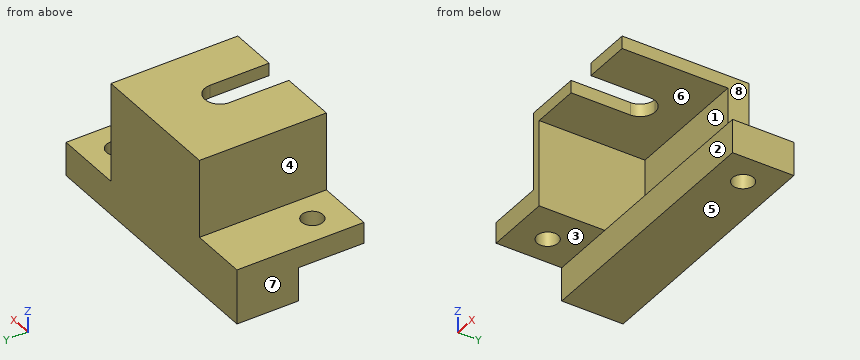
```python
from build123d import *

# Parameters (mm, degrees)
SKIZZE1_W                       = 24.6
SKIZZE1_H                       = 5.8
SKIZZE1_R                       = 1
AUFSATZ_LINEAR_AUSTRAGEN1_DEPTH = 3.2
SKIZZE2_W                       = 6.2
SKIZZE2_H                       = 12
AUFSATZ_LINEAR_AUSTRAGEN2_DEPTH = 2
SKIZZE3_R                       = 1
SCHNITT_LINEAR_AUSTRAGEN1_DEPTH = 2
AUFSATZ_LINEAR_AUSTRAGEN3_DEPTH = 8.2
SKIZZE5_W                       = 5.4
SKIZZE5_H                       = 1.2
AUFSATZ_LINEAR_AUSTRAGEN4_DEPTH = 12
SKIZZE6_W                       = 4.6
SKIZZE6_H                       = 8.2
SCHNITT_LINEAR_AUSTRAGEN2_DEPTH = 3.8
AUFSATZ_LINEAR_AUSTRAGEN5_DEPTH = 2.85
AUFSATZ_LINEAR_AUSTRAGEN6_DEPTH = 4.5
VERRUNDUNG1_R                   = 1.4


with BuildPart() as part:
    # Skizze1 → Aufsatz-Linear austragen1 (new body)
    with BuildSketch(Plane.XY):
        with Locations((12.3, 2.9)):
            Rectangle(SKIZZE1_W, SKIZZE1_H)
        with Locations((21.7, 2.9)):
            Circle(SKIZZE1_R, mode=Mode.SUBTRACT)
    extrude(amount=AUFSATZ_LINEAR_AUSTRAGEN1_DEPTH)

    # Skizze2 → Aufsatz-Linear austragen2 (add)
    with BuildSketch(Plane.XY.offset(3.2)):
        with Locations((3.1, -0.2)):
            Rectangle(SKIZZE2_W, SKIZZE2_H)
    extrude(amount=AUFSATZ_LINEAR_AUSTRAGEN2_DEPTH)

    # Skizze3 → Schnitt-Linear austragen1 (cut)
    with BuildSketch(Plane(origin=(0, 0, 3.2), x_dir=(-1, 0, 0), z_dir=(0, 0, -1))):
        with Locations((-2.7, -3.1)):
            Circle(SKIZZE3_R)
    extrude(amount=-SCHNITT_LINEAR_AUSTRAGEN1_DEPTH, mode=Mode.SUBTRACT)

    # Skizze4 → Aufsatz-Linear austragen3 (add)
    with BuildSketch(Plane.XY.offset(3.2)):
        Polygon((6.2, 5.8), (10.8, 5.8), (10.8, 0), (6.2, 0), (6.2, -6.2), (5.4, -6.2), (5.4, 5.8), align=None)
    extrude(amount=AUFSATZ_LINEAR_AUSTRAGEN3_DEPTH)

    # Skizze5 → Aufsatz-Linear austragen4 (add)
    with BuildSketch(Plane(origin=(0, 5.8, 0), x_dir=(1, 0, 0), z_dir=(0, 1, 0))):
        with Locations((8.1, -12)):
            Rectangle(SKIZZE5_W, SKIZZE5_H)
    extrude(amount=-AUFSATZ_LINEAR_AUSTRAGEN4_DEPTH)

    # Skizze6 → Schnitt-Linear austragen2 (cut)
    with BuildSketch(Plane.XZ):
        with Locations((8.5, 7.3)):
            Rectangle(SKIZZE6_W, SKIZZE6_H)
    extrude(amount=-SCHNITT_LINEAR_AUSTRAGEN2_DEPTH, mode=Mode.SUBTRACT)

    # Skizze7 → Aufsatz-Linear austragen5 (add)
    with BuildSketch(Plane(origin=(10.8, 0, 0), x_dir=(0, 0, -1), z_dir=(1, 0, 0))):
        Polygon((-12.6, 5.8), (-12.6, 0.8), (-11.4, 0.8), (-11.4, 3.8), (-3.2, 3.8), (-3.2, 5.8), align=None)
    extrude(amount=AUFSATZ_LINEAR_AUSTRAGEN5_DEPTH)

    # Skizze8 → Aufsatz-Linear austragen6 (add)
    with BuildSketch(Plane(origin=(13.65, 0, 0), x_dir=(0, 0, -1), z_dir=(1, 0, 0))):
        Polygon((-3.2, 5.8), (-12.6, 5.8), (-12.6, -6.2), (-11.4, -6.2), (-11.4, 3.8), (-3.2, 3.8), align=None)
    extrude(amount=AUFSATZ_LINEAR_AUSTRAGEN6_DEPTH)

    # Verrundung1
    verrundung1_edges = [part.edges().sort_by_distance(p)[0] for p in [
        (13.65, 0.8, 12),
        (10.8, 0.8, 12),
    ]]
    fillet(verrundung1_edges, radius=VERRUNDUNG1_R)


solid = part.part
```
Input: part model. Units: mm. Frame: model coordinates. Face numbers are marked on the shaded views. A direction names the side the tool comes from. Coordinates: 2 decimals unless noted, no trailing zeros. Write each loop counter-clockwise with the first axis right and the second up, starting at its lowest first coordinate (ties: lowest second). Pieces come first, ordered by that corner, then holes. Notation, with made-up numbers: (5, -17) -> (49, -17) arc R21 cw to (49, 18) -> close; hole circle Ø11 at (89, 55.25). An arc over 180 degrees is marked (long way). Answer as a JSON object with one key per item and string values.
1. Access query for the marked faces 4, 5, 6, 7 and 8. Directions: +Z, -Z, +X, -X, +Y, -Y. A direction counts if a zero-diameter tool reaches every point of the face in a straight line with its end or side. Return the directions, or none.
Result set:
{"face 4": "+Z, -X, +Y, -Y", "face 5": "-Z, +X, -X, +Y, -Y", "face 6": "+X, -Y", "face 7": "+Z, -Z, -X, +Y, -Y", "face 8": "+Z, +X, +Y, -Y"}
2. Section B-B on x = 2.7. Return the cut outline in (y, z).
Result set:
{"outline": "(-6.2, 3.2) -> (-4.1, 3.2) -> (-4.1, 5.2) -> (-6.2, 5.2) -> close; (-2.1, 3.2) -> (0, 3.2) -> (0, 0) -> (5.8, 0) -> (5.8, 5.2) -> (-2.1, 5.2) -> close"}
3. Section D-D on y = -3.1. Return the cut outline in (x, z).
Result set:
{"outline": "(0, 3.2) -> (1.7, 3.2) -> (1.7, 5.2) -> (0, 5.2) -> close; (3.7, 3.2) -> (6.2, 3.2) -> (6.2, 11.4) -> (10.8, 11.4) -> (10.8, 12.6) -> (5.4, 12.6) -> (5.4, 5.2) -> (3.7, 5.2) -> close; (13.65, 11.4) -> (18.15, 11.4) -> (18.15, 12.6) -> (13.65, 12.6) -> close"}
4. Section C-C on z = 3.5. Return the cut outline in (x, y), then the cut area to 3 significant figures.
Result set:
{"outline": "(0, -6.2) -> (6.2, -6.2) -> (6.2, 3.8) -> (18.15, 3.8) -> (18.15, 5.8) -> (0, 5.8) -> close; hole circle Ø2 at (2.7, -3.1)", "area": "95.2 mm2"}
5. First-contact query: P1, Ø1.3, axis at y = -3.5, z = 11.5, coming from the -X side; P2, Ø5, axis at y = -5, z = 3.5, coming from the +X side; P3, Ø4.5, axis at y = 3, z = 10, coming from the +X side; P4, Ø1.6, axis at x = 2.7, y = -3.1, coming from the +Z side. Flat tips, straight axial feed; report the tip coordinate or a pass-through.
Result set:
{"P1": "stops at x = 5.4", "P2": "stops at x = 6.2", "P3": "stops at x = 18.15", "P4": "passes through"}
6. Material intervals for line 1 (Z direction, x = 15.5, y = 2.5); line 2 (Y direction, x = 21.7, z = 0.85); line 3 (Y direction, x = 2.7, z = 4.1), sorted ascending. Write a range as from..to.
Result set:
{"line 1": "z = 0..3.2, 11.4..12.6", "line 2": "y = 0..1.9, 3.9..5.8", "line 3": "y = -6.2..-4.1, -2.1..5.8"}
7. Section A-A on y = 2.9. Return the cut outline in (x, z).
Result set:
{"outline": "(0, 0) -> (20.7, 0) -> (20.7, 3.2) -> (6.2, 3.2) -> (6.2, 11.4) -> (18.15, 11.4) -> (18.15, 12.6) -> (5.4, 12.6) -> (5.4, 5.2) -> (0, 5.2) -> close; (22.7, 0) -> (24.6, 0) -> (24.6, 3.2) -> (22.7, 3.2) -> close"}
8. Mould query, pull axis Z, two halves, no side actions, for the marked faces 1, 2 and 3. Classes: released by +Z, released by -Z, zero draft, split by the parting line, or undercut.
Result set:
{"face 1": "undercut", "face 2": "zero draft", "face 3": "released by -Z"}
